Check sheet for the modelled part. Datum: model origin and axes. Units: mm. A direction names the side the tool comes from. Round coordinates to 2 decimals unless told otherwise and drop trailing zeros. Loops run counter-clockwise (first coordinate to the right, second up) from the corner with the lowest first, then second, coordinate; pieces in that order, holes last. Notation, with made-up numbers: (23, -27) - (54, -27) arc R9 ccw to (54, -22) - close; hole circle Ø11 at (37, -11.5). An arc over 180 degrees is marked (long way). Answer in a Markdown table with one row per item. Add a question column.
(1) Cross-section at D-D on x = 6. Enter the section's corners in (y, z), then the cut area to 3 significant figures.
(2) Mould release check, pull along Z, two halves, no side actions. Record for faces 1 (the flat face through (13, 0, 52)), 2 (the flat face through (16, -10.5, 25)), 3 (the cylindrical face through (26.99, -0.69, 48.7)): +Z half, -Z half, draft (parallel to the pull), parting line (faces both ways), or undercut.
(3) Thickness scan on line 1 along Z through (x, y) = (12.5, 5.5); line 2 along Y through (x, z) = (6.5, 22) (3 decimals); line 3 along Z through (x, y) = (23.5, 12.5). Record the ranges inside material, lowest first.
(4) Gauge pin test, flat ends, axial feed: pin 1 (11 mm diameter, centred on x = -5.5, z = 23.5, fed in from +Y); pin 2 (3 mm diameter, centred on x = -5.5, y = 20, fed in from -Z); pin 3 (11 mm diameter, centred on x = -2, z = 38, fed in from -Y). Record the tip position at first contact, or that the pin passes through.
(5) Cross-section at C-C on x = 0. Enter the section's corners in (y, z).
(6) Access from +Z, -Z, +X, -X, +Y, -Y to the whole of each face (thin tool, end or side, straight path). Record for faces 4 (the flat face through (16, 10.5, 25)), 5 (the flat face through (-3, 19, 4.5)), 6 (the flat face through (15, -3.5, 2)), 7 (the flat face through (9, -21, 45.5)).
(7) Cross-section at B-B on z = 44. Enter the section's corners in (x, y).
(8) Cross-section at A-A on y = 0. Enter the section's corners in (x, z).
from build123d import *

# Parameters (mm, degrees)
CYLINDER091_R     = 21
CYLINDER091_DEPTH = 6.5
CYLINDER092_R     = 25
CYLINDER092_DEPTH = 6.5
BOX032_W          = 14
BOX032_H          = 50
BOX032_DEPTH      = 5.5
BOX031_W          = 14
BOX031_H          = 30
BOX031_DEPTH      = 53
BOX004_W          = 24
BOX004_H          = 7
BOX004_DEPTH      = 7
BOX003_W          = 55
BOX003_H          = 56
BOX003_DEPTH      = 71
BOX002_W          = 50
BOX002_H          = 21
BOX002_DEPTH      = 41
CYLINDER033_R     = 25
CYLINDER033_DEPTH = 53


with BuildPart() as cylinder091:
    # Cylinder091 → Cylinder091 (new body)
    with BuildSketch(Plane(origin=(6, 0, 45.5), x_dir=(1, 0, 0), z_dir=(0, 0, 1))):
        Circle(CYLINDER091_R)
    extrude(amount=CYLINDER091_DEPTH)


with BuildPart() as cut096:
    # Cylinder092 → Cylinder092 (new body)
    with BuildSketch(Plane(origin=(6, 0, 45.5), x_dir=(1, 0, 0), z_dir=(0, 0, 1))):
        Circle(CYLINDER092_R)
    extrude(amount=CYLINDER092_DEPTH)

    # Cut096: cut Cylinder091
    add(cylinder091.part, mode=Mode.SUBTRACT)


with BuildPart() as cube016:
    # Box032 → Box032 (new body)
    with BuildSketch(Plane(origin=(-11, -25, -1), x_dir=(1, 0, 0), z_dir=(0, 0, 1))):
        with Locations((7, 25)):
            Rectangle(BOX032_W, BOX032_H)
    extrude(amount=BOX032_DEPTH)


with BuildPart() as cube015:
    # Box031 → Box031 (new body)
    with BuildSketch(Plane(origin=(-11, -15, -1), x_dir=(1, 0, 0), z_dir=(0, 0, 1))):
        with Locations((7, 15)):
            Rectangle(BOX031_W, BOX031_H)
    extrude(amount=BOX031_DEPTH)


with BuildPart() as cube004:
    # Box004 → Box004 (new body)
    with BuildSketch(Plane(origin=(3, -3.5, -1), x_dir=(1, 0, 0), z_dir=(0, 0, 1))):
        with Locations((12, 3.5)):
            Rectangle(BOX004_W, BOX004_H)
    extrude(amount=BOX004_DEPTH)


with BuildPart() as cube003:
    # Box003 → Box003 (new body)
    with BuildSketch(Plane(origin=(-66, -25, -15), x_dir=(1, 0, 0), z_dir=(0, 0, 1))):
        with Locations((27.5, 28)):
            Rectangle(BOX003_W, BOX003_H)
    extrude(amount=BOX003_DEPTH)


with BuildPart() as cube002:
    # Box002 → Box002 (new body)
    with BuildSketch(Plane(origin=(-15, -10.5, 4.5), x_dir=(1, 0, 0), z_dir=(0, 0, 1))):
        with Locations((25, 10.5)):
            Rectangle(BOX002_W, BOX002_H)
    extrude(amount=BOX002_DEPTH)


with BuildPart() as cut097:
    # Cylinder033 → Cylinder033 (new body)
    with BuildSketch(Plane(origin=(6, 0, -1), x_dir=(1, 0, 0), z_dir=(0, 0, 1))):
        Circle(CYLINDER033_R)
    extrude(amount=CYLINDER033_DEPTH)

    # Cut026: cut Cube002
    add(cube002.part, mode=Mode.SUBTRACT)

    # Cut027: cut Cube003
    add(cube003.part, mode=Mode.SUBTRACT)

    # Cut028: cut Cube004
    add(cube004.part, mode=Mode.SUBTRACT)

    # Cut089: cut Cube015
    add(cube015.part, mode=Mode.SUBTRACT)

    # Cut090: cut Cube016
    add(cube016.part, mode=Mode.SUBTRACT)

    # Cut097: cut Cut096
    add(cut096.part, mode=Mode.SUBTRACT)


solid = cut097.part
Answers:
| question | item | result |
|---|---|---|
| 1 | outline | (-25, -1) - (-3.5, -1) - (-3.5, 4.5) - (-10.5, 4.5) - (-10.5, 45.5) - (10.5, 45.5) - (10.5, 4.5) - (3.5, 4.5) - (3.5, -1) - (25, -1) - (25, 45.5) - (21, 45.5) - (21, 52) - (-21, 52) - (-21, 45.5) - (-25, 45.5) - close |
| 1 | area | 1,700 mm^2 |
| 2 | face 1 | +Z half |
| 2 | face 2 | undercut |
| 2 | face 3 | draft |
| 3 | line 1 | z = -1 to 4.5, 45.5 to 52 |
| 3 | line 2 | y = -24.995 to -10.5, 10.5 to 24.995 |
| 3 | line 3 | z = -1 to 45.5 |
| 4 | pin 1 | stops at y = 24.27 |
| 4 | pin 2 | stops at z = 4.5 |
| 4 | pin 3 | stops at y = -24.87 |
| 5 | outline | (-24.27, 4.5) - (-15, 4.5) - (-15, 52) - (-20.12, 52) - (-20.12, 45.5) - (-24.27, 45.5) - close; (15, 4.5) - (24.27, 4.5) - (24.27, 45.5) - (20.12, 45.5) - (20.12, 52) - (15, 52) - close |
| 6 | face 4 | +X, -X |
| 6 | face 5 | -Z, -X, +Y, -Y |
| 6 | face 6 | -Z, -X |
| 6 | face 7 | +Z, -Y |
| 7 | outline | (-11, -18.33) arc R25 ccw to (28.69, -10.5) - (3, -10.5) - (3, -15) - (-11, -15) - close; (-11, 15) - (3, 15) - (3, 10.5) - (28.69, 10.5) arc R25 ccw to (-11, 18.33) - close |
| 8 | outline | (3, 45.5) - (27, 45.5) - (27, 52) - (3, 52) - close; (27, -1) - (31, -1) - (31, 4.5) - (27, 4.5) - close |
